from build123d import *

# Parameters (mm, degrees)
BOSS_EXTRUDE1_DEPTH = 16
CUT_EXTRUDE1_DEPTH  = 49.274320296
CUT_EXTRUDE2_START  = 6.4
CUT_EXTRUDE2_DEPTH  = 42.874320296
SKETCH4_R           = 3.298649114
CUT_EXTRUDE3_DEPTH  = 49.274320296


with BuildPart() as part:
    # Sketch1 → Boss-Extrude1 (new, symmetric)
    with BuildSketch(Plane.XY):
        Polygon((15.9, 0), (-18.9, 0), (-18.9, 16), (-22.5, 16), (-23.9, 14.650657895), (-27.9, 14.650657895), (-27.9, 21), (-18.9, 21), (-18.9, 36), (-13.4, 36), (15.9, 5.6), align=None)
    extrude(amount=BOSS_EXTRUDE1_DEPTH, both=True)

    # Sketch2 → Cut-Extrude1 (cut, through all)
    with BuildSketch(Plane.XZ):
        with BuildLine():
            Line((0, 16), (0, 22.397200509))
            Line((0, 22.397200509), (24.633267537, 22.397200509))
            Line((24.633267537, 22.397200509), (24.633267537, -22.936337669))
            Line((24.633267537, -22.936337669), (0, -22.936337669))
            Line((0, -22.936337669), (0, -16))
            ThreePointArc((0, -16), (16, 0), (0, 16))
        make_face()
    extrude(amount=-CUT_EXTRUDE1_DEPTH, mode=Mode.SUBTRACT)

    # Sketch3 → Cut-Extrude2 (cut, through all)
    with BuildSketch(Plane(origin=(0, 0, 0), x_dir=(1, 0, 0), z_dir=(0, 1, 0)).offset(CUT_EXTRUDE2_START)):
        with BuildLine():
            Line((-13.4, -12.4), (-13.4, 12.4))
            Line((-13.4, 12.4), (0, 12.4))
            ThreePointArc((0, 12.4), (8.193652125, 9.307204997), (12.3, 1.571623365))
            Line((12.3, 1.571623365), (12.3, -1.571623365))
            ThreePointArc((12.3, -1.571623365), (8.193652125, -9.307204997), (0, -12.4))
            Line((0, -12.4), (-13.4, -12.4))
        make_face()
    extrude(amount=CUT_EXTRUDE2_DEPTH, mode=Mode.SUBTRACT)

    # Sketch4 → Cut-Extrude3 (cut, through all)
    with BuildSketch(Plane(origin=(0, 0, 0), x_dir=(1, 0, 0), z_dir=(0, 1, 0))):
        with Locations(Location((0, 0, 0), (0, 0, 270))):
            Circle(SKETCH4_R)
    extrude(amount=CUT_EXTRUDE3_DEPTH, mode=Mode.SUBTRACT)


solid = part.part
CAD build for the part. Positions are in the model's coordinates, mm. A direction names the side the tool comes from. Round coordinates to 2 decimals unless told otherwise and drop trailing zeros. Write each loop counter-clockwise with the first axis right and the second up, starting at its lowest first coordinate (ties: lowest second). Pieces come first, ordered by that corner, then holes. Notation, with made-up numbers: M 45.5,19 L 84.5,19 A17 cw 84.5,27 Z; hole C 18.5,-12 d6. An arc over 180 degrees is marked long. Use a Markdown table: item, result. Add a question column.
1. Slice it at B-B on y = 2.5. Give the cut face in (x, z), then the cut area to 4 significant figures.
2. Slice it at C-C on y = 19.5. Give the cut face in (x, z).
3. Drill centre lines: probe 1 along X at (y, z) = (3, 0); probe 2 along Z at (x, y) = (-5, 25.5); probe 3 along X at (y, z) = (30.5, -1.5). Where is each one in solid material? Low to high.
4. Pull direction Y, two halves, no side cores. Call faces 1 (the face through (-26, 14.651, 0)), 2 (the face through (4.44, 17.49, -11.78)), 3 (the face through (-27.9, 18, 0)): released by +Y, released by -Y, zero draft, split by the parting line, or undercut.
5. 3-axis set-ups, long thin cutter, end or side, ignore diameter. For faces 4 (the face through (-11, 14, -16)), 5 (the face through (-7, 18, 12.4)), 6 (the face through (-23, 21, 0)): which of +Z, -Z, +X, -X, +Y, -Y reach the whole face in a straight line?
6. Slice it at D-D on x = 9.5. Give the cut face in (y, z), then the cut area to 3 significant figures.
7. Slice it at A-A on z = 0. Give the cut face in (x, y).
8. Flat gauge pins, fed straight in: P1, Ø8, axis at y = 3.5, z = -11.5, coming from the +X side; P2, Ø2, axis at x = -9, z = -11, coming from the +Y side; P3, Ø4.5, axis at x = -22.5, z = -5, coming from the +Y side; P4, Ø12, axis at x = -20, y = 32.5, coming from the +Z side. Where does each tip first touch, or does it go through?
Reply:
| question | item | result |
|---|---|---|
| 1 | outline | M -18.9,-16 L 0,-16 A16 ccw 15.9,-1.79 L 15.9,1.79 A16 ccw 0,16 L -18.9,16 Z; hole C 0,0 d6.6 |
| 1 | area | 972.5 mm^2 |
| 2 | outline | M -27.9,-16 L 0,-16 A16 ccw 2.5,-15.8 L 2.5,-12.14 A12.4 cw 0,-12.4 L -13.4,-12.4 L -13.4,12.4 L 0,12.4 A12.4 cw 2.5,12.14 L 2.5,15.8 A16 ccw 0,16 L -27.9,16 Z |
| 3 | probe 1 | x = -18.9 to -3.3, 3.3 to 15.9 |
| 3 | probe 2 | z = -16 to -12.4, 12.4 to 16 |
| 3 | probe 3 | x = -18.9 to -13.4 |
| 4 | face 1 | released by -Y |
| 4 | face 2 | released by +Y |
| 4 | face 3 | zero draft |
| 5 | face 4 | -Z, +X, -X, +Y, -Y |
| 5 | face 5 | +Y |
| 5 | face 6 | +Z, -Z, -X, +Y |
| 6 | outline | M 0,-12.87 L 12.24,-12.87 L 12.24,-7.97 L 6.4,-7.97 L 6.4,7.97 L 12.24,7.97 L 12.24,12.87 L 0,12.87 Z |
| 6 | area | 222 mm^2 |
| 7 | outline | M -27.9,14.65 L -23.9,14.65 L -22.5,16 L -18.9,16 L -18.9,0 L -3.3,0 L -3.3,6.4 L -13.4,6.4 L -13.4,36 L -18.9,36 L -18.9,21 L -27.9,21 Z; M 3.3,0 L 15.9,0 L 15.9,5.6 L 12.3,9.34 L 12.3,6.4 L 3.3,6.4 Z |
| 8 | P1 | stops at x = 14.13 |
| 8 | P2 | stops at y = 6.4 |
| 8 | P3 | stops at y = 21 |
| 8 | P4 | stops at z = 16 |
